The drawing under review shows one solid part. Ordinate dimensions are in mm from its lowest x, y, z. Give positions to 0.01 mm unless a question says otherwise; leave off trailing zeros. Write each loop counter-clockwise with the first axis right and the second up, starting at its lowest first coordinate (ties: lowest second). Pieces come first, ordered by that corner, then holes. Notation, with made-up numbers: M 84.25,38 L 101.25,38 A14 cw 101.25,56 Z; hole C 34.5,37.5 d11. An arc over 180 degrees is marked long. Write item = value, one per line. Start each with the question number.
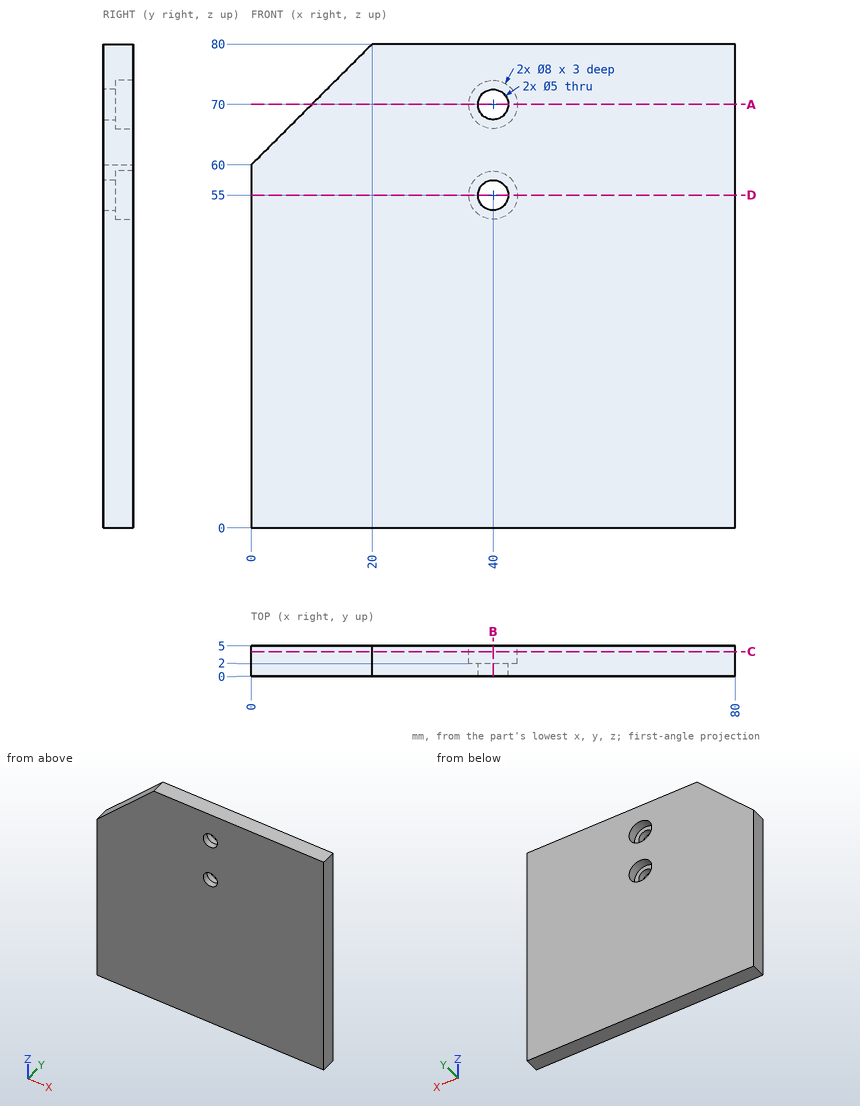
Item 1: Clearance check with a flat-ended pin moving along its axis: P1, Ø6.5, axis at x = 38.5, z = 69.5, coming from the +Y side. State where the tip first meets the part, or that it passes through.
Item 2: To check wall thickness, follow probe 1 along X at (y, z) = (2.8, 55); probe 2 along X at (y, z) = (0.8, 65); probe 3 along X at (y, z) = (2.6, 70). State the ranges of each line that lie inside material, in increasing order. Write a range as [from, to].
Item 3: We need section B-B, the plane x = 40. Write out the cut boundary in (y, z), and give its area (3 significant figures).
Item 4: We need section D-D, the plane z = 55. Write out the cut boundary in (x, y).
Item 5: We need section C-C, the plane y = 4.05. Write out the cut boundary in (x, z), and give its area (3 significant figures).
Item 6: We need section A-A, the plane z = 70. Write out the cut boundary in (x, y).
Worked out:
q1.P1 = 5
q2.probe_1 = [0, 36], [44, 80]
q2.probe_2 = [5, 80]
q2.probe_3 = [10, 36], [44, 80]
q3.outline = M 0,0 L 5,0 L 5,51 L 2,51 L 2,52.5 L 0,52.5 Z; M 0,57.5 L 2,57.5 L 2,59 L 5,59 L 5,66 L 2,66 L 2,67.5 L 0,67.5 Z; M 0,72.5 L 2,72.5 L 2,74 L 5,74 L 5,80 L 0,80 Z
q3.area = 332 mm²
q4.outline = M 0,0 L 37.5,0 L 37.5,2 L 36,2 L 36,5 L 0,5 Z; M 42.5,0 L 80,0 L 80,5 L 44,5 L 44,2 L 42.5,2 Z
q5.outline = M 0,0 L 80,0 L 80,80 L 20,80 L 0,60 Z; hole C 40,55 d8; hole C 40,70 d8
q5.area = 6,100 mm²
q6.outline = M 10,0 L 37.5,0 L 37.5,2 L 36,2 L 36,5 L 10,5 Z; M 42.5,0 L 80,0 L 80,5 L 44,5 L 44,2 L 42.5,2 Z
